Could you check a few things on this model? Use its own coordinates, in mm. A direction names the side the tool comes from. Give positions to 0.01 mm unless a question says otherwise; leave off trailing zeros. Loops run counter-clockwise (first coordinate to the right, second up) from the corner with the lowest first, then second, coordinate; pieces in that order, holes last. Notation, with made-up numbers: (88.5, -35.75) - (94.5, -35.75) arc R8 cw to (94.5, -21.75) - close; hole circle Ø9 at (86.5, 71.5). An arc over 180 degrees is marked (long way). Write each question's results on one line, items separated by ' | '. Start each with the question number.
(1) Suppose I cut it at D-D (x = 13). Please give me the cut outline in (y, z).
(2) For pin 1 (3.5 mm diameter, centred on x = 1.5, y = -5.5, fed in from -Z); pin 2 (4.5 mm diameter, centred on x = -30.5, z = -30.5, fed in from -Y); pin 3 (2 mm diameter, centred on y = -4.5, z = -36.5, fed in from -X), each with a flat end and sliding along its axis, tell me the tip position at first contact or that it passes through.
(3) Suppose I cut it at A-A (x = -22.5). Please give me the cut outline in (y, z), and give its area (3 significant figures).
(4) I need wall thicknesses on line 1 (Z direction, x = -17, y = -0.75) (3 decimals); line 2 (X direction, y = -5, z = -37.05); line 3 (Y direction, x = 0, z = 37). Which ranges of each line are inside material? Lowest first, please.
(5) If we mould it in two halves opening along Z, with no side actions, what happens to faces 5 (the face through (-29, -4, 33)), 6 (the face through (-35, 0, -1)), 7 (the face through (2, 1, -42))? For each: released by +Z, released by -Z, zero draft, split by the parting line, or undercut.
(6) Suppose I cut it at B-B (z = -13). Please give me the cut outline in (x, y), and give its area (3 significant figures).
(7) On a 3-axis mill with a long thin cutter (end or side, diameter ignored), from which of +Z, -Z, +X, -X, +Y, -Y can I reach the whole of each face in a straight line? I mean faces 1 (the face through (-2.5, -5, -37)), 2 (the face through (-20.05, 0, -14)), 3 (the face through (-31, -4, 15)), 4 (the face through (-31, -4, -19)). Say none if no direction works.
(8) Suppose I cut it at C-C (z = 7). Please give me the cut outline in (x, y).
from build123d import *

# Parameters (mm, degrees)
SKETCH009_W             = 84
SKETCH009_H             = 70
PAD002_DEPTH            = 2
SKETCH010_W             = 2
SKETCH010_H             = 7
PAD003_DEPTH            = 2
SKETCH012_W             = 8
SKETCH012_H             = 6.8
PAD004_DEPTH            = 4
SKETCH013_W             = 7
SKETCH013_H             = 6
PAD005_DEPTH            = 4
SKETCH011_W             = 8
SKETCH011_H             = 6.8
PAD006_DEPTH            = 4
SKETCH014_R             = 1.15
POCKET002_DEPTH         = 81.001
SKETCH016_R             = 1.15
POCKET003_DEPTH         = 8.501
SKETCH018_W             = 11.5
SKETCH018_H             = 11.5
POCKET004_DEPTH         = 5
POCKET005_DEPTH         = 5
POCKET006_DEPTH         = 5
SKETCH021_W             = 1
SKETCH021_H             = 7
PAD007_DEPTH            = 1
SKETCH022_W             = 9
SKETCH022_H             = 10
POCKET007_DEPTH         = 0.4
FILLET_R                = 3
BODY002_PITCH_ANGLE     = -90
BODY002_PLACEMENT_ANGLE = 90
PAD001_DEPTH            = 35
SKETCH007_W             = 11.5
SKETCH007_H             = 11.5
POCKET001_DEPTH         = 13
FILLET001_R             = 3
SKETCH025_W             = 6.5
SKETCH025_H             = 9
SKETCH025_W_2           = 9
SKETCH025_H_2           = 6.5
POCKET008_DEPTH         = 8


with BuildPart() as back:
    # Sketch009 → Pad002 (new body)
    with BuildSketch(Plane.XY):
        Rectangle(SKETCH009_W, SKETCH009_H)
    extrude(amount=PAD002_DEPTH)

    # Sketch010 (on Face6 of Pad002) → Pad003 (join)
    with BuildSketch(Plane.XY.offset(2)):
        with Locations((-38, -1)):
            Rectangle(SKETCH010_W, SKETCH010_H)
        Polygon((-21, 32), (39, 32), (39, -4), (37, -4), (37, 30), (-21, 30), align=None)
    extrude(amount=PAD003_DEPTH)

    # Sketch012 (on Face15 of Pad003) → Pad004 (join)
    with BuildSketch(Plane.YZ.offset(39)):
        with Locations((0, 5.4)):
            Rectangle(SKETCH012_W, SKETCH012_H)
    extrude(amount=-PAD004_DEPTH)

    # Sketch013 (on Face9 of Pad004) → Pad005 (join)
    with BuildSketch(Plane(origin=(-39, 0, 0), x_dir=(0, -1, 0), z_dir=(-1, 0, 0))):
        with Locations((1, 5)):
            Rectangle(SKETCH013_W, SKETCH013_H)
    extrude(amount=-PAD005_DEPTH)

    # Sketch011 (on Face16 of Pad003) → Pad006 (join)
    with BuildSketch(Plane(origin=(0, 32, 0), x_dir=(-1, 0, 0), z_dir=(0, 1, 0))):
        with Locations((-29, 5.4)):
            Rectangle(SKETCH011_W, SKETCH011_H)
        with Locations((14, 5.4)):
            Rectangle(SKETCH011_W, SKETCH011_H)
    extrude(amount=-PAD006_DEPTH)

    # Sketch014 (on Face44 of Pad006) → Pocket002 (cut, through all)
    with BuildSketch(Plane.YZ.offset(39)):
        with Locations((0, 5)):
            Circle(SKETCH014_R)
    extrude(amount=-POCKET002_DEPTH, mode=Mode.SUBTRACT)

    # Sketch016 → Pocket003 (cut, through all)
    with BuildSketch(Plane.XZ.offset(-26.5)):
        with Locations((-13, 5)):
            Circle(SKETCH016_R)
        with Locations((30, 5)):
            Circle(SKETCH016_R)
    extrude(amount=-POCKET003_DEPTH, mode=Mode.SUBTRACT)

    # Sketch018 (on Face5 of Pocket003) → Pocket004 (cut)
    with BuildSketch(Plane.XY.offset(2)):
        with Locations((0, 17.75)):
            Rectangle(SKETCH018_W, SKETCH018_H)
    extrude(amount=-POCKET004_DEPTH, mode=Mode.SUBTRACT)

    # Sketch019 (on Face31 of Pocket004) → Pocket005 (cut)
    with BuildSketch(Plane.XZ.offset(-28)):
        Polygon((29.125944, 9.042901), (33.258869, 4.499726), (33.258869, 9.042901), align=None)
    extrude(amount=-POCKET005_DEPTH, mode=Mode.SUBTRACT)

    # Sketch020 (on Face36 of Pocket005) → Pocket006 (cut)
    with BuildSketch(Plane(origin=(35, 0, 0), x_dir=(0, -1, 0), z_dir=(-1, 0, 0))):
        Polygon((2.77547, 8.938441), (6.386171, 3.079567), (6.386171, 8.938441), align=None)
    extrude(amount=-POCKET006_DEPTH, mode=Mode.SUBTRACT)

    # Sketch021 (on Face40 of Pocket006) → Pad007 (join)
    with BuildSketch(Plane.XY.offset(8)):
        with Locations((-38.5, -1)):
            Rectangle(SKETCH021_W, SKETCH021_H)
    extrude(amount=PAD007_DEPTH)

    # Sketch022 (on Face5 of Pocket005) → Pocket007 (cut)
    with BuildSketch(Plane.XY.offset(2)):
        with Locations((-30.3, 30)):
            Rectangle(SKETCH022_W, SKETCH022_H)
    extrude(amount=-POCKET007_DEPTH, mode=Mode.SUBTRACT)

    # Fillet
    fillet_edges = [back.edges().sort_by_distance(p)[0] for p in [
        (42, 35, 1),
        (-42, 35, 1),
    ]]
    fillet(fillet_edges, radius=FILLET_R)


with BuildPart() as back_1:
    # Body002 pitch: moved
    add(back.part.rotate(Axis((0, 0, 0), (0, 1, 0)), BODY002_PITCH_ANGLE))


with BuildPart() as back_2:
    # Body002 placement: moved
    add(back_1.part.rotate(Axis((0, 0, 0), (0, 0, 1)), BODY002_PLACEMENT_ANGLE))


with BuildPart() as curve:
    # Sketch006 → Pad001 (new body, symmetric)
    with BuildSketch(Plane(origin=(0, 0, 0), x_dir=(0, 0, -1), z_dir=(1, 0, 0))):
        with BuildLine():
            ThreePointArc((-42, 3.9), (0, 0.511678), (42, 3.9))
            Line((42, -0.1), (42, 3.9))
            Line((-42, -0.1), (42, -0.1))
            Line((-42, 3.9), (-42, -0.1))
        make_face()
    extrude(amount=PAD001_DEPTH, both=True)

    # Sketch007 (on Face3 of Pad001) → Pocket001 (cut)
    with BuildSketch(Plane.XZ.offset(0.1)):
        with Locations((-17.75, 0)):
            Rectangle(SKETCH007_W, SKETCH007_H)
    extrude(amount=-POCKET001_DEPTH, mode=Mode.SUBTRACT)

    # Fillet001
    fillet001_edges = [curve.edges().sort_by_distance(p)[0] for p in [
        (-35, 1.9, -42),
        (-35, 1.9, 42),
    ]]
    fillet(fillet001_edges, radius=FILLET001_R)

    # Boolean: union Back
    add(back_2.part)

    # Sketch025 (on Face32 of Boolean) → Pocket008 (cut, symmetric)
    with BuildSketch(Plane.XZ.offset(2)):
        with Locations((-28.75, 0)):
            Rectangle(SKETCH025_W, SKETCH025_H)
        with Locations((-15.55, 13.625)):
            Rectangle(SKETCH025_W_2, SKETCH025_H_2)
        with Locations((-2.05, 0)):
            Rectangle(SKETCH025_W, SKETCH025_H)
        with Locations((-15.55, -13.625)):
            Rectangle(SKETCH025_W_2, SKETCH025_H_2)
    extrude(amount=POCKET008_DEPTH, both=True, mode=Mode.SUBTRACT)


solid = curve.part
Output values:
1) outline: (-2, -42) - (3.9, -42) arc R262 cw to (3.9, 42) - (-2, 42) - close
2) pin 1: z = -39 | pin 2: y = -1.6 | pin 3: x = -2.5
3) outline: (-4, 37) - (-2, 37) - (-2, 5.75) - (0.57, 5.75) arc R262 cw to (3.9, 42) - (-2, 42) - (-2, 39) - (-4, 39) - close; (-2, -42) - (3.9, -42) arc R262 cw to (0.57, -5.75) - (-2, -5.75) - close | area: 280 mm2
4) line 1: -42 to -16.875, -10.375 to -5.75, 5.75 to 10.375, 16.875 to 42 | line 2: -2.5 to -1.15, 1.15 to 4.5 | line 3: -8.8 to -6.15, -3.85 to 3.14
5) face 5: undercut | face 6: zero draft | face 7: released by -Z
6) outline: (-35, -2) - (-32, -2) - (-32, -3.85) - (-28, -3.85) - (-28, -2) - (-20.05, -2) - (-20.05, 0.83) - (-35, 0.83) - close; (-32, -8.8) - (-28, -8.8) - (-28, -6.15) - (-32, -6.15) - close; (-11.05, -2) - (35, -2) - (35, 0.83) - (-11.05, 0.83) - close | area: 191 mm2
7) face 1: -Z, -X, -Y | face 2: +Y, -Y | face 3: +X, -X, -Y | face 4: -Z, +X, -X, -Y
8) outline: (-35, -2) - (-32, -2) - (-32, -4) - (-30, -4) - (-30, -2) - (35, -2) - (35, 0.61) - (-35, 0.61) - close
